Autodesk Inventor part; units mm, degrees
ref_plane "YZ Plane" through (0, 0, 0) normal (1, 0, 0) x (0, 1, 0)
ref_plane "XZ Plane" through (0, 0, 0) normal (0, 1, 0) x (-1, 0, 0)
ref_plane "XY Plane" through (0, 0, 0) normal (0, 0, 1) x (1, 0, 0)
sketch "Sketch1" plane through (0, 0, 0) normal (0, 0, 1) x (1, 0, 0)
  line L0 (-29, 60) -> (29, 60)
  line L1 (15, 60) -> (-15, 60)
  line L2 (-15, 60) -> (-15, 55)
  line L3 (-15, 55) -> (15, 55)
  line L4 (15, 55) -> (15, 60)
  point P0 (0, 0)
  point P1 (-15, 60)
  dimension "d0" = 5
  dimension "d1" = 15
  dimension "d2" = 15
extrude "Extrusion1" add sketch "Sketch1" along normal blind 20
sketch "Sketch2" plane through (-15, 60, 0) normal (0, 1, 0) x (1, 0, 0)
  circle A0 centre (19.75, -15) radius 1.5
  circle A1 centre (10.25, -15) radius 1.5
  line L0 (30, -20) -> (0, -20)
  line L1 (0, 0) -> (0, -20)
  point P0 (15, 0)
  dimension "d5" = 9.5
  dimension "d6" = 5
  dimension "d7" = 5
  dimension "d8" = 10.25
  dimension "d9" = 3
  dimension "d10" = 3
hole "Hole1" at (4.75, 60, 15) at (-4.75, 60, 15) direction (0, -1, 0) diameter 3 depth 20 tip angle 118
fillet "Fillet1" radius 5 2 edges at (15, 57.5, 20) (-15, 57.5, 20)
sketch "Sketch3" plane through (0, 0, 0) normal (0, 0, -1) x (-1, 0, 0)
  circle A0 centre (-8.5, 57.5001) radius 1.5
  circle A1 centre (8.5, 57.5) radius 1.5
  point P0 (0, 0)
hole "Hole2" at (8.5, 57.5001, 0) at (-8.5, 57.5, 0) direction (0, 0, 1) diameter 2.459 depth 20 tip angle 118
equation "\"d11\" = d10"
properties part number "Z-Endstophalter1"
The listing builds one solid part. Answer for the finished solid, in the listing's coordinates (mm). Give positions to 0.01 mm unless a question says otherwise; leave off trailing zeros. Order: outer loops, then holes, each group sorted by start corner. A loop starts at its lowest first (then second) coordinate and runs counter-clockwise, first axis right, second up. Notation, with made-up numbers: (76.25, 24.25) -> (88.25, 24.25) arc R11 ccw to (88.25, 29.25) -> close; hole circle Ø5 at (76, 22). An arc over 180 degrees is marked (long way). Answer as a JSON object with one key per item and string values. Group by question number.
Item 1: Consider L1, parallel to X at y = 57.5, z = 15; L2, parallel to Y at x = -8.5, z = 7; L3, parallel to Z at x = -4.75, y = 57.7. Determine where each line is inside the solid, lowest interval first. Write a range as from..to.
Item 2: The part is cut by section C-C on z = 8.5. Write down the section's boundary in (x, y), and give its area (3 significant figures).
Item 3: The part is cut by section A-A on x = -8.5. Write down the section's boundary in (y, z).
Item 4: The part is cut by section B-B on y = 57.5. Write down the section's boundary in (x, z), and give its area (3 significant figures).
Item 5: Determine the mould class of faces 1 (the cylindrical face through (-8.55, 56.27, 10.14)), 2 (the flat face through (-15, 58, 7)), 3 (the cylindrical face through (8.971, 58.636, 10.14)), 4 (the flat face through (0, 55, 10)) for opening direction Y: pulls with the +Y half, pulls with the -Y half, needs draft (parallel to the pull), parting line crosses it, or undercut.
Item 6: Flat-ended cylindrical pins translate along their axes: pin 1 (3 mm diameter, centred on x = 8.5, y = 57.5, fed in from +Z); pin 2 (2.5 mm diameter, centred on x = 4.75, z = 15, fed in from +Y). Find the tip coordinate at first contact, or state that the pin passes through.
Item 7: The part is cut by section D-D on x = 4.75. Write down the section's boundary in (y, z).
Result set:
{
 "1": {"L1": "-15..-9.73, -7.27..-6.25, -3.25..3.25, 6.25..7.27, 9.73..15", "L2": "55..56.27, 58.73..60", "L3": "0..13.5, 16.5..20"},
 "2": {"outline": "(-15, 55) -> (15, 55) -> (15, 60) -> (-15, 60) -> close; hole circle Ø2.46 at (-8.5, 57.5); hole circle Ø2.46 at (8.5, 57.5)", "area": "141 mm²"},
 "3": {"outline": "(55, 0) -> (56.27, 0) -> (56.27, 20) -> (55, 20) -> close; (58.73, 0) -> (60, 0) -> (60, 20) -> (58.73, 20) -> close"},
 "4": {"outline": "(-15, 0) -> (-9.73, 0) -> (-9.73, 20) -> (-10, 20) arc R5 ccw to (-15, 15) -> close; (-7.27, 0) -> (7.27, 0) -> (7.27, 20) -> (-7.27, 20) -> close; (9.73, 0) -> (15, 0) -> (15, 15) arc R5 ccw to (10, 20) -> (9.73, 20) -> close; hole circle Ø3 at (-4.75, 15); hole circle Ø3 at (4.75, 15)", "area": "477 mm²"},
 "5": {"face 1": "undercut", "face 2": "needs draft", "face 3": "undercut", "face 4": "pulls with the -Y half"},
 "6": {"pin 1": "z = 20", "pin 2": "through"},
 "7": {"outline": "(55, 0) -> (60, 0) -> (60, 13.5) -> (55, 13.5) -> close; (55, 16.5) -> (60, 16.5) -> (60, 20) -> (55, 20) -> close"}
}
